Here's how the part is built. I have some questions about the finished solid (model axes, mm). A direction names the side the tool comes from. Round coordinates to 2 decimals unless told otherwise and drop trailing zeros. Loops run counter-clockwise (first coordinate to the right, second up) from the corner with the lowest first, then second, coordinate; pieces in that order, holes last. Notation, with made-up numbers: M 16,-10.5 L 34,-10.5 A14 ccw 34,7.5 Z; hole C -23.75,59 d3. An arc over 180 degrees is marked long. Put each result on its own line as item: value. Start each with the question number.
```python
from build123d import *

# Parameters (mm, degrees)
F1_DEPTH      = 65
F2_R          = 155
F3_DEPTH      = 55
F4_W          = 22.4599032382
F4_H          = 50
F5_DEPTH      = 65.001
F5_DEPTH_BACK = 65.001


with BuildPart() as f1:
    # F0 (on Right) → F1 (new body, symmetric)
    with BuildSketch(Plane.YZ):
        with BuildLine():
            Line((0, 49.1090789437), (0, 0))
            Line((0, 0), (6.4133200794, 0))
            Line((6.4133200794, 0), (6.4133200794, 33.1709496677))
            Line((6.4133200794, 33.1709496677), (12.8133200794, 33.1709496677))
            Line((12.8133200794, 33.1709496677), (12.8133200794, 0))
            Line((12.8133200794, 0), (27.3600688376, 0))
            Line((27.3600688376, 0), (133.5539043449, 166.1648069956))
            ThreePointArc((133.5539043449, 166.1648069956), (81.4380712008, 152.1940833921), (62.8215606058, 202.8366219893))
            Line((62.8215606058, 202.8366219893), (0, 49.1090789437))
        make_face()
        with BuildLine():
            ThreePointArc((139.8490899801, 187.705129385), (107.5594344934, 226.9549776329), (62.8215606058, 202.8366219893))
            ThreePointArc((62.8215606058, 202.8366219893), (81.4380712008, 152.1940833921), (133.5539043449, 166.1648069956))
            ThreePointArc((133.5539043449, 166.1648069956), (138.2430515795, 176.4844470214), (139.8490899801, 187.705129385))
        make_face()
    extrude(amount=F1_DEPTH, both=True)

    # F2 (on Right) → F3 (cut, symmetric)
    with BuildSketch(Plane.YZ):
        with Locations((100, 200)):
            Circle(F2_R)
    extrude(amount=F3_DEPTH, both=True, mode=Mode.SUBTRACT)

    # F4 (on Right) → F5 (cut, two sides)
    with BuildSketch(Plane.YZ) as f5_sk:
        with Locations((100, 215.2752558307)):
            Rectangle(F4_W, F4_H)
    extrude(amount=-F5_DEPTH, mode=Mode.SUBTRACT)
    extrude(f5_sk.sketch, amount=F5_DEPTH_BACK, mode=Mode.SUBTRACT)


solid = f1.part
```
1) If I drill on probe 1 along X at (y, z) = (83, 129); probe 2 along Z at (x, y) = (-59.5, 8.5); probe 3 along Z at (x, y) = (25.5, 47.5), over which ranges is the centre line in solid material (lowest first)? Write a range as from..to.
2) I'm going to push flat-ended pins straight in: P1, Ø5, axis at x = 59, z = 214.5, coming from the -Y side; P2, Ø5, axis at x = -59, z = 201.5, coming from the +Y side; P3, Ø8, axis at x = 60, z = 210.5, coming from the +Y side. Where does each tip first touch, or does it pass through?
3) If we mould it in two halves opening along X, with no side actions, what happens to faces 4 (the face through (60, 88.77, 208)), 5 (the face through (65, 69, 115)), 6 (the face through (0.77, 33.42, 60.03))? For each: pulls with the +X half, pulls with the -X half, needs draft (parallel to the pull), parting line crosses it, or undercut.
4) Suppose I cut it at A-A (z = 22.5). Write out the boundary of the cut face in (x, y), plus the area to 3 significant figures.
5) On a 3-axis mill with a long thin cutter (end or side, diameter ignored), from which of +Z, -Z, +X, -X, +Y, -Y can I reach the whole of each face in a straight line? I mean faces 1 (the face through (0.3, 8.29, 69.4)), 2 (the face through (1, 6.413, 16)), 3 (the face through (60, 100, 190.275)). Say none if no direction works.
6) Suppose I cut it at B-B (y = 82.5). Write out the boundary of the cut face in (x, z), plus the area to 3 significant figures.
7) Suppose I cut it at C-C (x = 12). Write out the boundary of the cut face in (y, z), plus the area to 3 significant figures.
8) Suppose I cut it at D-D (z = 208.5). Write out the boundary of the cut face in (x, y).
Results are:
1. probe 1: -65..-55, 55..65
1. probe 2: 33.17..69.91
1. probe 3: 31.51..54.16
2. P1: y = 68.07
2. P2: y = 138.22
2. P3: y = 135.16
3. face 4: needs draft
3. face 5: pulls with the +X half
3. face 6: undercut
4. outline: M -65,0 L 65,0 L 65,6.41 L -65,6.41 Z; M -65,12.81 L 65,12.81 L 65,41.74 L -65,41.74 Z
4. area: 4,590 mm²
5. face 1: +Z, +X, -X, -Y
5. face 2: -Z, +X, -X
5. face 3: +Z, +X, -X
6. outline: M -65,86.28 L -55,86.28 L -55,223.75 L -65,223.75 Z; M 55,86.28 L 65,86.28 L 65,223.75 L 55,223.75 Z
6. area: 2,750 mm²
7. outline: M 0,0 L 6.41,0 L 6.41,33.17 L 12.81,33.17 L 12.81,0 L 27.36,0 L 59.55,50.37 A155 cw 10.07,73.75 L 0,49.11 Z
7. area: 2,580 mm²
8. outline: M -65,65.68 L -55,65.68 L -55,88.77 L -65,88.77 Z; M -65,111.23 L -55,111.23 L -55,134.02 L -65,134.02 Z; M 55,65.68 L 65,65.68 L 65,88.77 L 55,88.77 Z; M 55,111.23 L 65,111.23 L 65,134.02 L 55,134.02 Z
